Part model, mm, in its own coordinate system. Give positions to 0.01 mm unless a question says otherwise; leave off trailing zeros. Write each loop counter-clockwise with the first axis right and the second up, starting at its lowest first coordinate (ties: lowest second). Pieces come first, ordered by that corner, then holes. Notation, with made-up numbers: M -7.75,67 L 25.25,67 A29 ccw 25.25,104 Z; hole C -32,54 d5. An arc over 180 degrees is marked long. Use a Markdown table: item, result.
```python
from build123d import *

# Parameters (mm, degrees)
CROQUIS1_W              = 24
CROQUIS1_H              = 144
SALIENTE_EXTRUIR1_DEPTH = 20
CORTAR_EXTRUIR2_DEPTH   = 148.349923651
CROQUIS4_W              = 24
CROQUIS4_H              = 70


with BuildPart() as part:
    # Croquis1 → Saliente-Extruir1 (new body)
    with BuildSketch(Plane(origin=(0, 0, 0), x_dir=(1, 0, 0), z_dir=(0, 1, 0))):
        with Locations((12, 72)):
            Rectangle(CROQUIS1_W, CROQUIS1_H)
    extrude(amount=SALIENTE_EXTRUIR1_DEPTH)

    # Croquis3 → Cortar-Extruir2 (cut, through all)
    with BuildSketch(Plane(origin=(24, 0, 0), x_dir=(0, 0, -1), z_dir=(1, 0, 0))):
        Polygon((144, 20), (0, 0), (0, 20), align=None)
    extrude(amount=-CORTAR_EXTRUIR2_DEPTH, mode=Mode.SUBTRACT)

    # Croquis4 → Cortar-Revolución2 (revolve, cut)
    with BuildSketch(Plane.XZ):
        with Locations((12, -109)):
            Rectangle(CROQUIS4_W, CROQUIS4_H)
    revolve(axis=Axis((0, 0, 0), (1, 0, 0)), mode=Mode.SUBTRACT)


with BuildPart() as body_2:
    # of the pieces the cut leaves, the one that is kept (cortar_revoluci_n2_keep)
    add(part.part.solids().sort_by_distance((0, 0, -74))[0])


solid = body_2.part
```
1. Drop flat-ended pins along their axis: P1, Ø10, axis at x = 6, z = -35.5, coming from the +Y side (3 decimals); P2, Ø2, axis at y = 8.5, z = -42.5, coming from the -X side; P3, Ø3, axis at x = 12, z = -8.5, coming from the +Y side; P4, Ø2, axis at x = 9.5, z = -33, coming from the +Y side. Give the stop position or say it passes through.
Findings below:
| item | result |
|---|---|
| P1 | y = 5.625 |
| P2 | through |
| P3 | y = 1.39 |
| P4 | y = 4.72 |
2. Drill centre lines: L1, parallel to Y at x = 10.25, z = -66; L2, parallel to Y at x = 16.5, z = -29. Where is each one in solid material? Low to high.
Findings below:
| item | result |
|---|---|
| L1 | 0 to 9.17 |
| L2 | 0 to 4.03 |
3. Cut at C-C, the plane z = -18. Give the cut face in (x, y).
Findings below:
| item | result |
|---|---|
| outline | M 0,0 L 24,0 L 24,2.5 L 0,2.5 Z |
4. Cut at B-B, the plane y = 5. Give the cut face in (x, z).
Findings below:
| item | result |
|---|---|
| outline | M 0,-73.83 L 24,-73.83 L 24,-36 L 0,-36 Z |
5. Cut at A-A, the plane x = 22.25. Give the cut face in (y, z).
Findings below:
| item | result |
|---|---|
| outline | M 0,-74 A74 ccw 10.18,-73.3 L 0,0 Z |
